from build123d import *

# Parameters (mm, degrees)
F0_R     = 245
F0_R_2   = 2.5
F0_R_3   = 150
F0_W     = 25
F0_H     = 10
F1_DEPTH = 25


with BuildPart() as f1:
    # F0 (on Front) → F1 (new body)
    with BuildSketch(Plane.XZ):
        Circle(F0_R)
        with Locations((-137.8858223314, -137.8858223314)):
            Circle(F0_R_2, mode=Mode.SUBTRACT)
        with Locations((-130.8147545195, -130.8147545195)):
            Circle(F0_R_2, mode=Mode.SUBTRACT)
        with Locations((137.8858223314, -137.8858223314)):
            Circle(F0_R_2, mode=Mode.SUBTRACT)
        with Locations((130.8147545195, -130.8147545195)):
            Circle(F0_R_2, mode=Mode.SUBTRACT)
        with Locations((-130.8147545195, 130.8147545195)):
            Circle(F0_R_2, mode=Mode.SUBTRACT)
        with Locations((-137.8858223314, 137.8858223314)):
            Circle(F0_R_2, mode=Mode.SUBTRACT)
        Circle(F0_R_3, mode=Mode.SUBTRACT)
        Polygon((40, 205), (40, 165), (-40, 165), (-40, 205), (-12.5, 205), (-12.5, 215), (12.5, 215), (12.5, 205), align=None, mode=Mode.SUBTRACT)
        with Locations((130.8147545195, 130.8147545195)):
            Circle(F0_R_2, mode=Mode.SUBTRACT)
        with Locations((137.8858223314, 137.8858223314)):
            Circle(F0_R_2, mode=Mode.SUBTRACT)
        with Locations((0, 210)):
            Rectangle(F0_W, F0_H)
    extrude(amount=F1_DEPTH)


solid = f1.part
Can you work these out from the model? Positions are in its coordinate system, mm. A direction names the side the tool comes from. Give positions to 0.01 mm unless a question says otherwise; leave off trailing zeros. Loops run counter-clockwise (first coordinate to the right, second up) from the corner with the lowest first, then second, coordinate; pieces in that order, holes last. Notation, with made-up numbers: (-39.75, 1) - (-31.75, 1) arc R30 cw to (-31.75, 24) - close; hole circle Ø2 at (-8.75, 21). An arc over 180 degrees is marked (long way). One line per item, written item: value.
(1) If we section it at D-D, the plane z = -111.5: List the corners of the cut face in (x, y) for me, plus the area to 3 significant figures.
Verdict:
outline: (-218.16, -25) - (-100.34, -25) - (-100.34, 0) - (-218.16, 0) - close; (100.34, -25) - (218.16, -25) - (218.16, 0) - (100.34, 0) - close
area: 5,890 mm^2
(2) I'm going to push flat-ended pins straight in: pin 1 (5 mm diameter, centred on x = -19.5, y = -21, fed in from -Z); pin 2 (4 mm diameter, centred on x = 174, y = -21.5, fed in from -Z); pin 3 (3 mm diameter, centred on x = 137.89, z = 137.89, fed in from -Y); pin 4 (2 mm diameter, centred on y = -12, z = -39, fed in from +X). Where does each tip first touch, or does it pass through?
Verdict:
pin 1: z = -244.41
pin 2: z = -174.47
pin 3: through
pin 4: x = 242.04
(3) If we mould it in two halves opening along Z, with no side actions, what happens to faces 3 (the face through (1, -12, 165)), 4 (the face through (-3, 0, -160)), 5 (the face through (-53.111, -12.325, -239.174))? For each: released by +Z, released by -Z, zero draft, split by the parting line, or undercut.
Verdict:
face 3: undercut
face 4: zero draft
face 5: split by the parting line
(4) If we section it at B-B, the plane x = 0: List the corners of the cut face in (y, z) for me.
Verdict:
outline: (-25, -245) - (0, -245) - (0, -150) - (-25, -150) - close; (-25, 150) - (0, 150) - (0, 165) - (-25, 165) - close; (-25, 205) - (0, 205) - (0, 245) - (-25, 245) - close
(5) If we section it at C-C, the plane y = -4: State how many separate pieces and enclosed holes the cut face has, plus the area to 3 significant figures.
Verdict:
separate pieces: 1
enclosed holes: 10
area: 115,000 mm^2
(6) I need wall thicknesses on line 1 along Z through (x, y) = (-8.5, -3.75); line 2 along Z through (x, y) = (31.5, -8.25); line 3 along Z through (x, y) = (137, -13.5). Which ranges of each line are inside material? Lowest first, please.
Verdict:
line 1: -244.85 to -149.76, 149.76 to 165, 205 to 244.85
line 2: -242.97 to -146.66, 146.66 to 165, 205 to 242.97
line 3: -203.12 to -140.22, -135.55 to -61.08, 61.08 to 135.55, 140.22 to 203.12
(7) If we section it at A-A, the plane z = 0: List the corners of the cut face in (x, y) for me.
Verdict:
outline: (-245, -25) - (-150, -25) - (-150, 0) - (-245, 0) - close; (150, -25) - (245, -25) - (245, 0) - (150, 0) - close
(8) On a 3-axis mill with a long thin cutter (end or side, diameter ignored), from which of +Z, -Z, +X, -X, +Y, -Y can I reach the whole of each face in a straight line? I mean faces 1 (the face through (-40, -12, 185)), 2 (the face through (-3, -25, -160)). Say none if no direction works.
Verdict:
face 1: +Y, -Y
face 2: +Z, -Z, +X, -X, -Y
